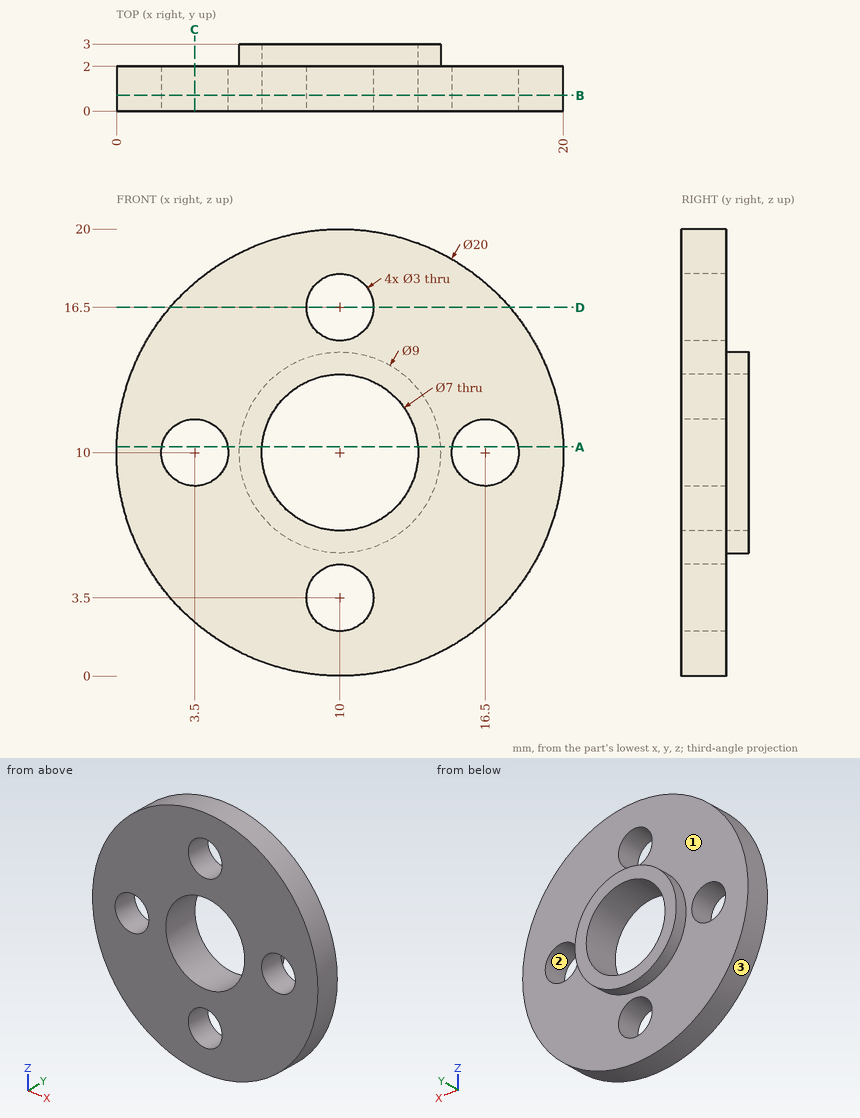
Print and shaded views of the part. All mm, measured from the part's lowest x, y and z. Coordinates: 2 decimals unless noted, no trailing zeros. Loops run counter-clockwise (first coordinate to the right, second up) from the corner with the lowest first, then second, coordinate; pieces in that order, holes last. Notation, with made-up numbers: (23, -8.5) - (71, -8.5) arc R30 ccw to (71, 21.5) - close; hole circle Ø11 at (-34.75, 72.25). An arc over 180 degrees is marked (long way). Write item = value, one per line. Start each with the question number.
Item 1: Wall check: probe 1 along X at (y, z) = (0.6, 10); probe 2 along Z at (x, y) = (9.5, 1.65). Give the ranges that are in metal, low to high. Write a range as [from, to].
Item 2: Drop flat-ended pins along their axis: pin 1 Ø1.5 at (y, z) = (1, 14) entering from +X; pin 2 Ø3.5 at (x, z) = (10, 3.5) entering from +Y; pin 3 Ø1 at (x, y) = (15, 2) entering from -Z. Give the stop position or say it passes through.
Item 3: Pull direction X, two halves, no side cores. Call the marked faces 1, 2 and 3: +X half, -X half, draft (parallel to the pull), parting line (faces both ways), or undercut.
Item 4: Saw through at B-B, the plane y = 0.7. List the corners of the cut face in (x, z).
Item 5: Saw through at D-D, the plane z = 16.5. List the corners of the cut face in (x, y), then the cut area to 3 significant figures.
Item 6: Saw through at C-C, the plane x = 3.5. List the corners of the cut face in (y, z).
Item 7: Saw through at A-A, the plane z = 10.25. List the corners of the cut face in (x, y), then the cut area to 3 significant figures.
Answers:
q1.probe_1 = [0, 2], [5, 6.5], [13.5, 15], [18, 20]
q1.probe_2 = [0.01, 2.09], [4.91, 6.54], [13.46, 15.09], [17.91, 19.99]
q2.pin_1 = 19.46
q2.pin_2 = 2
q2.pin_3 = 1.07
q3.face_1 = draft
q3.face_2 = undercut
q3.face_3 = parting line
q4.outline = circle Ø20 at (10, 10); hole circle Ø3 at (3.5, 10); hole circle Ø7 at (10, 10); hole circle Ø3 at (10, 3.5); hole circle Ø3 at (10, 16.5); hole circle Ø3 at (16.5, 10)
q5.outline = (2.4, 0) - (8.5, 0) - (8.5, 2) - (2.4, 2) - close; (11.5, 0) - (17.6, 0) - (17.6, 2) - (11.5, 2) - close
q5.area = 24.4 mm2
q6.outline = (0, 2.4) - (2, 2.4) - (2, 8.5) - (0, 8.5) - close; (0, 11.5) - (2, 11.5) - (2, 17.6) - (0, 17.6) - close
q7.outline = (0, 0) - (2.02, 0) - (2.02, 2) - (0, 2) - close; (4.98, 0) - (6.51, 0) - (6.51, 3) - (5.51, 3) - (5.51, 2) - (4.98, 2) - close; (13.49, 0) - (15.02, 0) - (15.02, 2) - (14.49, 2) - (14.49, 3) - (13.49, 3) - close; (17.98, 0) - (20, 0) - (20, 2) - (17.98, 2) - close
q7.area = 16.2 mm2
